Here's how the part is built. I have some questions about the finished solid (model axes, mm). A direction names the side the tool comes from. Coordinates: 2 decimals unless noted, no trailing zeros. Loops run counter-clockwise (first coordinate to the right, second up) from the corner with the lowest first, then second, coordinate; pieces in that order, holes last. Notation, with made-up numbers: (-7.75, 83.5) - (33.25, 83.5) arc R30 ccw to (33.25, 108.5) - close; hole circle Ø11 at (1, -24). An arc over 180 degrees is marked (long way). Use a Markdown table: item, result.
```python
from build123d import *

# Parameters (mm, degrees)
SKETCH2_R          = 3.175
CUT_EXTRUDE1_DEPTH = 2.54
CIRPATTERN1_COUNT  = 8


with BuildPart() as part:
    # Sketch1 → Revolve1 (revolve)
    with BuildSketch(Plane.XY):
        Polygon((0, 31.75), (24.13, 39.878), (24.13, 76.2), (48.26, 76.2), (48.26, 101.6), (45.72, 101.6), (45.72, 78.74), (21.59, 78.74), (21.59, 41.702647785), (-0.810815928, 34.157109788), align=None)
    revolve(axis=Axis((0, 0, 0), (1, 0, 0)))

    # Sketch2 → Cut-Extrude1 (cut)
    with BuildSketch(Plane.ZY.offset(-45.72)):
        with Locations((0, 85.09)):
            Circle(SKETCH2_R)
    cut_extrude1 = extrude(amount=-CUT_EXTRUDE1_DEPTH, mode=Mode.SUBTRACT)

    # CirPattern1: Cut-Extrude1 ×8 about axis
    cirpattern1_axis = Axis((0, 0, 0), (1, 0, 0))
    for i in range(1, CIRPATTERN1_COUNT):
        add(cut_extrude1.rotate(cirpattern1_axis, i * 360 / CIRPATTERN1_COUNT), mode=Mode.SUBTRACT)


solid = part.part
```
Q1. I want a section at B-B, the plane z = 85.09. Write out the boundary of the cut face in (x, y) (3 decimals).
Check values:
| item | result |
|---|---|
| outline | (45.72, -55.518) - (48.26, -55.518) - (48.26, -3.175) - (45.72, -3.175) - close; (45.72, 3.175) - (48.26, 3.175) - (48.26, 55.518) - (45.72, 55.518) - close |
Q2. Will these pins go through, and if not, where does the flat tip stop? P1, Ø10, axis at y = 60.17, z = -60.17, coming from the -X side; P2, Ø2, axis at x = 33.5, y = 16.5, coming from the +Z side; P3, Ø1, axis at x = 19, z = 23, coming from the +Y side.
Check values:
| item | result |
|---|---|
| P1 | x = 45.72 |
| P2 | z = 77.2 |
| P3 | y = 34.13 |
Q3. I want a section at D-D, the plane y = -51.5. Write out the boundary of the cut face in (x, z), then the cut area to 3 significant figures.
Check values:
| item | result |
|---|---|
| outline | (21.59, -59.56) - (45.72, -59.56) - (45.72, -87.58) - (48.26, -87.58) - (48.26, -56.16) - (24.13, -56.16) - (24.13, 56.16) - (48.26, 56.16) - (48.26, 87.58) - (45.72, 87.58) - (45.72, 59.56) - (21.59, 59.56) - close |
| area | 609 mm^2 |
Q4. Which directions (+Z, -Z, +X, -X, +Y, -Y) give clear straight access to the entire face, cutting with the end or side of a thin tool? Please do faces 1 (the face through (33.486, -62.485, -47.912)), 2 (the face through (46.972, -22.025, -99.184)), 3 (the face through (36.364, -60.47, -46.367)).
Check values:
| item | result |
|---|---|
| face 1 | -X |
| face 2 | +X, -X |
| face 3 | +X |
Q5. Please list where these lines run through material, in increasing order: L1, parallel to Z at x = 47.3, y = 0 (3 decimals); L2, parallel to Z at x = 32, y = 0; L3, parallel to X at y = -46, z = 33. Write a range as from..to.
Check values:
| item | result |
|---|---|
| L1 | -101.6..-88.265, -81.915..-76.2, 76.2..81.915, 88.265..101.6 |
| L2 | -78.74..-76.2, 76.2..78.74 |
| L3 | 21.59..24.13 |
Q6. I want a section at A-A, the plane z = 0. Write out the boundary of the cut face in (x, y) (3 decimals).
Check values:
| item | result |
|---|---|
| outline | (-0.811, -34.157) - (21.59, -41.703) - (21.59, -78.74) - (45.72, -78.74) - (45.72, -81.915) - (48.26, -81.915) - (48.26, -76.2) - (24.13, -76.2) - (24.13, -39.878) - (0, -31.75) - close; (-0.811, 34.157) - (0, 31.75) - (24.13, 39.878) - (24.13, 76.2) - (48.26, 76.2) - (48.26, 81.915) - (45.72, 81.915) - (45.72, 78.74) - (21.59, 78.74) - (21.59, 41.703) - close; (45.72, -101.6) - (48.26, -101.6) - (48.26, -88.265) - (45.72, -88.265) - close; (45.72, 88.265) - (48.26, 88.265) - (48.26, 101.6) - (45.72, 101.6) - close |
